```python
from build123d import *

# Parameters (mm, degrees)
SKETCH1_W           = 15
SKETCH1_H           = 11
BOSS_EXTRUDE1_DEPTH = 3.5
FILLET1_R           = 1
SKETCH2_W           = 12.7
SKETCH2_H           = 8.7
CUT_EXTRUDE1_DEPTH  = 0.5
FILLET2_R           = 2.55


with BuildPart() as part:
    # Sketch1 → Boss-Extrude1 (new body)
    with BuildSketch(Plane(origin=(0, 0, 0), x_dir=(1, 0, 0), z_dir=(0, 1, 0))):
        Rectangle(SKETCH1_W, SKETCH1_H)
    extrude(amount=BOSS_EXTRUDE1_DEPTH)

    # Fillet1
    fillet1_edges = [part.edges().sort_by_distance(p)[0] for p in [
        (7.5, 1.75, 5.5),
        (-7.5, 1.75, 5.5),
        (-7.5, 1.75, -5.5),
        (7.5, 1.75, -5.5),
    ]]
    fillet(fillet1_edges, radius=FILLET1_R)

    # Sketch2 → Cut-Extrude1 (cut)
    with BuildSketch(Plane(origin=(0, 3.5, 0), x_dir=(1, 0, 0), z_dir=(0, 1, 0))):
        Rectangle(SKETCH2_W, SKETCH2_H)
    extrude(amount=-CUT_EXTRUDE1_DEPTH, mode=Mode.SUBTRACT)

    # Fillet2
    fillet2_edges = [part.edges().sort_by_distance(p)[0] for p in [
        (6.35, 3.25, -4.35),
        (6.35, 3.25, 4.35),
        (-6.35, 3.25, 4.35),
        (-6.35, 3.25, -4.35),
    ]]
    fillet(fillet2_edges, radius=FILLET2_R)


solid = part.part
```
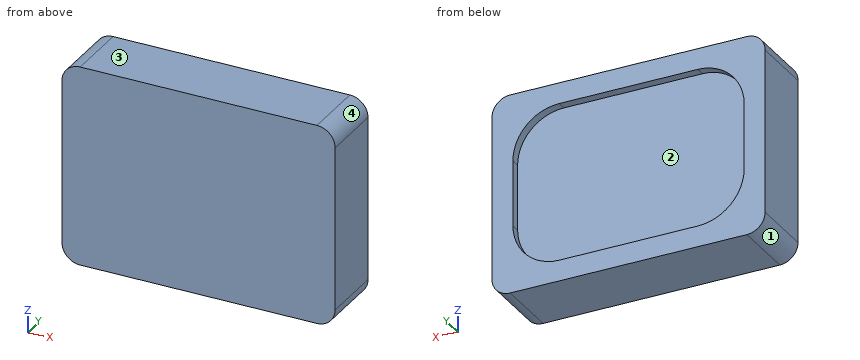
Here's how the part is built. I have some questions about the finished solid (model axes, mm). Face numbers are marked on the shaded views. Give positions to 0.01 mm unless a question says otherwise; leave off trailing zeros. Order: outer loops, then holes, each group sorted by start corner. A loop starts at its lowest first (then second) coordinate and runs counter-clockwise, first axis right, second up. Notation, with made-up numbers: (50.25, -25.5) - (83.25, -25.5) arc R30 ccw to (83.25, 6.5) - close; hole circle Ø4 at (28, 29.5). An arc over 180 degrees is marked (long way). Answer as a JSON object with one key per item and string values. Group by question number.
Item 1: For P1, Ø2.5, axis at x = 1.5, z = 1, coming from the +Y side, with a flat end and sliding along its axis, tell me the tip position at first contact or that it passes through.
Item 2: If we section it at C-C on z = 0.25: Please give me the cut outline in (x, y), and give its area (4 significant figures).
Item 3: If we section it at B-B on x = 0.25: Please give me the cut outline in (y, z).
Item 4: If we section it at A-A on y = 3.25: Please give me the cut outline in (x, z), and give its area (3 significant figures).
Item 5: Please list where these lines run through material, in increasing order: probe 1 along X at (y, z) = (3.3, -1.75); probe 2 along Y at (x, z) = (-2.75, -4).
Item 6: If we mould it in two halves opening along X, with no side actions, what happens to the marked faces 1, 2, 3 and 4? For each: pulls with the +X half, pulls with the -X half, needs draft (parallel to the pull), parting line crosses it, or undercut.
Result set:
{
 "1": {"P1": "y = 3"},
 "2": {"outline": "(-7.5, 0) - (7.5, 0) - (7.5, 3.5) - (6.35, 3.5) - (6.35, 3) - (-6.35, 3) - (-6.35, 3.5) - (-7.5, 3.5) - close", "area": "46.15 mm²"},
 "3": {"outline": "(0, -5.5) - (3.5, -5.5) - (3.5, -4.35) - (3, -4.35) - (3, 4.35) - (3.5, 4.35) - (3.5, 5.5) - (0, 5.5) - close"},
 "4": {"outline": "(-7.5, -4.5) arc R1 ccw to (-6.5, -5.5) - (6.5, -5.5) arc R1 ccw to (7.5, -4.5) - (7.5, 4.5) arc R1 ccw to (6.5, 5.5) - (-6.5, 5.5) arc R1 ccw to (-7.5, 4.5) - close; hole (-6.35, -1.8) arc R2.55 ccw to (-3.8, -4.35) - (3.8, -4.35) arc R2.55 ccw to (6.35, -1.8) - (6.35, 1.8) arc R2.55 ccw to (3.8, 4.35) - (-3.8, 4.35) arc R2.55 ccw to (-6.35, 1.8) - close", "area": "59.2 mm²"},
 "5": {"probe 1": "-7.5 to -6.35, 6.35 to 7.5", "probe 2": "0 to 3"},
 "6": {"face 1": "pulls with the -X half", "face 2": "undercut", "face 3": "needs draft", "face 4": "pulls with the +X half"}
}
